For this review, take the finished solid that the model builds, in its own axes (mm). A direction names the side the tool comes from. Give positions to 0.01 mm unless a question says otherwise; leave off trailing zeros. Loops run counter-clockwise (first coordinate to the right, second up) from the corner with the lowest first, then second, coordinate; pieces in that order, holes last. Notation, with made-up numbers: (45, 89.5) - (86, 89.5) arc R18 ccw to (86, 106.5) - close; hole circle Ø1 at (-20.75, 66.5). An arc over 180 degrees is marked (long way). Put each result on its own line as item: value.
from build123d import *

# Parameters (mm, degrees)
SKETCH1_R           = 19.5
BOSS_EXTRUDE1_DEPTH = 1
SKETCH2_R           = 18.5
BOSS_EXTRUDE2_DEPTH = 33
SKETCH3_R           = 19.5
BOSS_EXTRUDE3_DEPTH = 1
FILLET1_R           = 0.2
CHAMFER1_SIZE       = 0.2
SKETCH4_R           = 2.05
CUT_EXTRUDE1_DEPTH  = 45.558949718


with BuildPart() as part:
    # Sketch1 → Boss-Extrude1 (new body)
    with BuildSketch(Plane.XY):
        Circle(SKETCH1_R)
    extrude(amount=BOSS_EXTRUDE1_DEPTH)

    # Sketch2 → Boss-Extrude2 (add)
    with BuildSketch(Plane.XY.offset(1)):
        Circle(SKETCH2_R)
    extrude(amount=BOSS_EXTRUDE2_DEPTH)

    # Sketch3 → Boss-Extrude3 (add)
    with BuildSketch(Plane.XY.offset(34)):
        Circle(SKETCH3_R)
    extrude(amount=BOSS_EXTRUDE3_DEPTH)

    # Fillet1
    fillet1_edges = [part.edges().sort_by_distance(p)[0] for p in [
        (-18.5, 0, 1),
        (-18.5, 0, 34),
    ]]
    fillet(fillet1_edges, radius=FILLET1_R)

    # Chamfer1
    chamfer1_edges = [part.edges().sort_by_distance(p)[0] for p in [
        (-19.5, 0, 35),
        (-19.5, 0, 0),
        (-19.5, 0, 1),
        (-19.5, 0, 34),
    ]]
    chamfer(chamfer1_edges, length=CHAMFER1_SIZE)

    # Sketch4 → Cut-Extrude1 (cut, through all)
    with BuildSketch(Plane.XY.offset(35)):
        Circle(SKETCH4_R)
    extrude(amount=-CUT_EXTRUDE1_DEPTH, mode=Mode.SUBTRACT)


solid = part.part
1) Draft analysis for pull direction X (two halves, no side actions). For faces 3 (the face through (-0.267, 2.033, 17.745)), 4 (the face through (-2.539, 19.334, 0.496)), 5 (the face through (0, -4, 0)), state which applies: pulls with the +X half, pulls with the -X half, needs draft (parallel to the pull), parting line crosses it, or undercut.
Geometry check:
face 3: undercut
face 4: parting line crosses it
face 5: needs draft
2) Take a section at A-A on x = 0. State the section outline as (y, z) points, and give its area (3 significant figures).
Geometry check:
outline: (-19.5, 0.2) - (-19.3, 0) - (-2.05, 0) - (-2.05, 35) - (-19.3, 35) - (-19.5, 34.8) - (-19.5, 34.2) - (-19.3, 34) - (-18.7, 34) arc R0.2 cw to (-18.5, 33.8) - (-18.5, 1.2) arc R0.2 cw to (-18.7, 1) - (-19.3, 1) - (-19.5, 0.8) - close; (2.05, 0) - (19.3, 0) - (19.5, 0.2) - (19.5, 0.8) - (19.3, 1) - (18.7, 1) arc R0.2 cw to (18.5, 1.2) - (18.5, 33.8) arc R0.2 cw to (18.7, 34) - (19.3, 34) - (19.5, 34.2) - (19.5, 34.8) - (19.3, 35) - (2.05, 35) - close
area: 1,160 mm²
3) Wall thickness on line 1 (Y direction, x = 0, z = 23.5); line 2 (Z direction, x = 13.5, y = -14); line 3 (X direction, y = -3, z = 27.5): over which ranges is each line inside the solid? List them lowest first.
Geometry check:
line 1: y = -18.5 to -2.05, 2.05 to 18.5
line 2: z = 0.15 to 0.85, 34.15 to 34.85
line 3: x = -18.26 to 18.26
4) For faces 1 (the face through (-2.539, 19.334, 34.496)), 2 (the face through (-10, 16, 34)), list the 3-axis set-ups (+Z, -Z, +X, -X, +Y, -Y) from which the entire face can be reached by the end or side of a thin tool; tool diameter is ignored.
Geometry check:
face 1: +Z, -Z
face 2: none
5) Take a section at C-C on z = 7.5. State the section outline as (x, y) points.
Geometry check:
outline: circle Ø37 at (0, 0); hole circle Ø4.1 at (0, 0)
6) Insertion check: pin 1 Ø3 at (y, z) = (-8.5, 25) entering from +X; pin 2 Ø5 at (x, z) = (6, 10.5) entering from +Y; pin 3 Ø4 at (x, z) = (12, 30.5) entering from +Y. Each pin has a flat end and moves straight along its axis. Give the tip position at first contact, or say it passes through.
Geometry check:
pin 1: stops at x = 17.12
pin 2: stops at y = 18.17
pin 3: stops at y = 15.56
